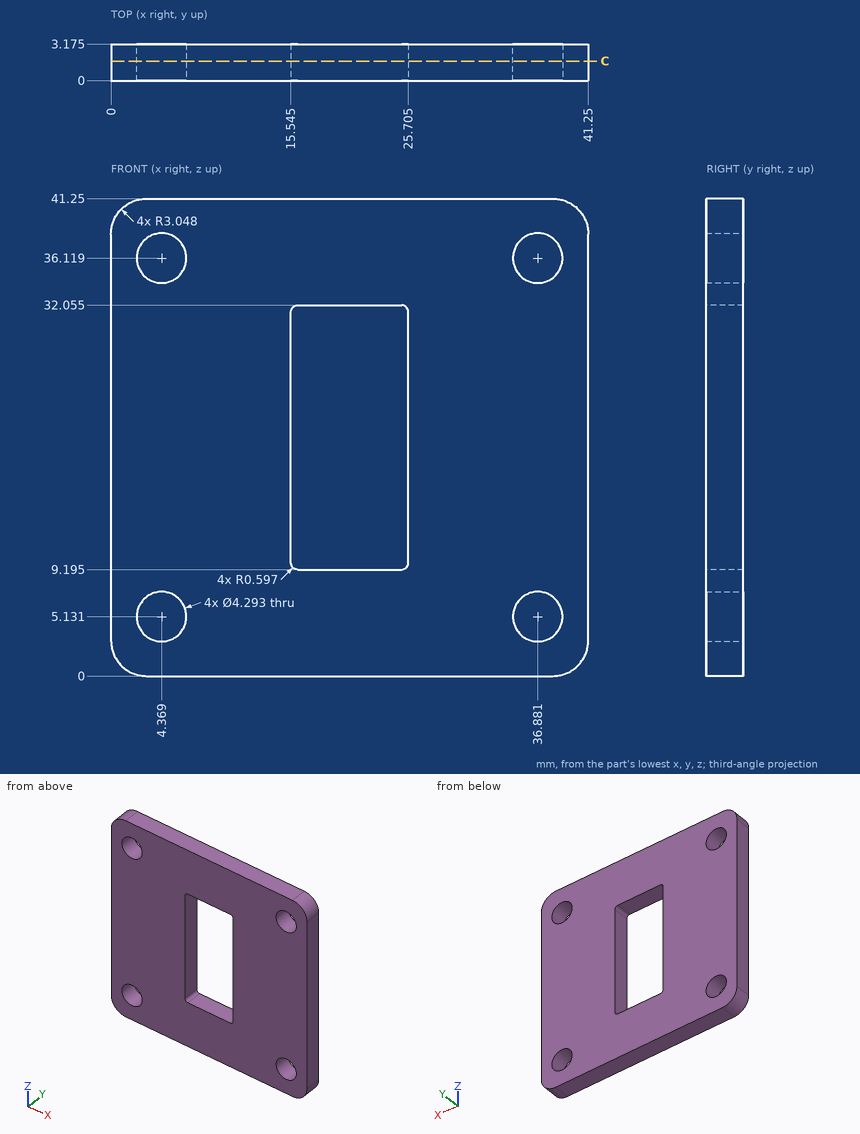
Drawing for the job (mm, zero at the part's lowest x, y, z). Give positions to 0.01 mm unless a question says otherwise; leave off trailing zeros. Write item = value, one per line. Start each with the question number.
(1) Pin check, flat tip, straight feed: pin 1 Ø2.5 at (x, z) = (36.88, 36.12) entering from -Y. Stop position of the tip, or through.
(2) Probe L1, parallel to Z at x = 38.5, y = 1.95 (1 decimal); L2, parallel to Z at x = 25.5, y = 1.2. List the from-to ranges inside material, lowest first. Write a range as [from, to].
(3) Slice it at C-C on y = 1.7. State how many separate pieces and enclosed holes the cut face has, plus the area to 3 significant figures.
Responses:
q1.pin_1 = through
q2.L1 = [0, 3.7], [6.5, 34.7], [37.5, 41.2]
q2.L2 = [0, 9.34], [31.91, 41.25]
q3.separate_pieces = 1
q3.enclosed_holes = 5
q3.area = 1,400 mm2
